from build123d import *

# Parameters (mm, degrees)
F0_R     = 33.04
F1_DEPTH = 58
F2_SIZE  = 7.62
F3_T     = -2.54
F4_R     = 2.54
F5_R     = 6
F5_W     = 10.6
F5_H     = 5
F6_DEPTH = 2.54
F7_W     = 35
F7_H     = 2.54
F8_DEPTH = 47
F9_R     = 2.54


with BuildPart() as f1:
    # F0 (on Top) → F1 (new body)
    with BuildSketch(Plane.XY):
        Circle(F0_R)
    extrude(amount=F1_DEPTH)

    # F2
    f2_edges = [f1.edges().sort_by_distance(p)[0] for p in [
        (-33.04, 0, 0),
    ]]
    chamfer(f2_edges, length=F2_SIZE)

    # F3
    f3_openings = [f1.faces().sort_by_distance(p)[0] for p in [
        (0, 0, 58),
    ]]
    offset(amount=F3_T, openings=f3_openings)

    # F4
    f4_edges = [f1.edges().sort_by_distance(p)[0] for p in [
        (-33.04, 0, 7.62),
        (-25.42, 0, 0),
    ]]
    fillet(f4_edges, radius=F4_R)

    # F5 (on face) → F6 (cut, through all)
    with BuildSketch(Plane(origin=(0, 0, 0), x_dir=(1, 0, 0), z_dir=(0, 0, -1))):
        with Locations((0, 7.62)):
            Circle(F5_R)
        with Locations((0, -6.35)):
            Rectangle(F5_W, F5_H)
    extrude(amount=-F6_DEPTH, mode=Mode.SUBTRACT)

    # F7 (on face) → F8 (join)
    with BuildSketch(Plane.XY.offset(2.54)):
        with Locations((0, 18.58)):
            Rectangle(F7_W, F7_H)
    extrude(amount=F8_DEPTH)

    # F9
    f9_edges = [f1.edges().sort_by_distance(p)[0] for p in [
        (-17.5, 18.58, 49.54),
        (17.5, 18.58, 49.54),
    ]]
    fillet(f9_edges, radius=F9_R)


solid = f1.part
Part model, mm, in its own coordinate system. A direction names the side the tool comes from. Coordinates: 2 decimals unless noted, no trailing zeros. Order: outer loops, then holes, each group sorted by start corner. A loop starts at its lowest first (then second) coordinate and runs counter-clockwise, first axis right, second up.
(1) Probe L1, parallel to Y at x = 0, z = 37; L2, parallel to X at y = 0, z = 35; L3, parallel to Y at x = 0, z = 1. List the from-to ranges inside material, lowest first.
Check sheet entries:
L1: y = -33.04 to -30.5, 17.31 to 19.85, 30.5 to 33.04
L2: x = -33.04 to -30.5, 30.5 to 33.04
L3: y = -26.42 to -13.62, -1.62 to 3.85, 8.85 to 26.42
(2) Tool access for faces 1 (the face through (0, 3.85, 1)), 2 (the face through (16.736, 18.598, 48.816)), 3 (the face through (0, 0, 0)): list every direction of +Z, -Z, +X, -X, +Y, -Y with a clear straight run to the whole face (end or side of a thin tool).
Check sheet entries:
face 1: +Z, -Z
face 2: +Z
face 3: -Z, +X, -X, +Y, -Y
(3) Pin check, flat tips, straight feed: pin 1 Ø2 at (x, y) = (-5.5, 19) entering from +Z; pin 2 Ø6 at (x, z) = (6.5, 16.5) entering from -Y; pin 3 Ø1.3 at (y, z) = (6.5, 1) entering from +X; pin 4 Ø11 at (x, y) = (0, -7.62) entering from +Z. Stop position of each tip, or through.
Check sheet entries:
pin 1: stops at z = 49.54
pin 2: stops at y = -32.85
pin 3: stops at x = 26.3
pin 4: passes through
(4) Pull direction X, two halves, no side cores. Call faces 4 (the face through (29, -10, 58)), 5 (the face through (-5.7, -25.8, 1)), 6 (the face through (0, 22, 2.54)): pulls with the +X half, pulls with the -X half, needs draft (parallel to the pull), parting line crosses it, or undercut.
Check sheet entries:
face 4: needs draft
face 5: parting line crosses it
face 6: undercut
(5) Slice it at A-A, the plane z = 46. Write the cut outline in (x, y).
Check sheet entries:
outline: circle Ø66.08 at (0, 0); (-17.5, 17.31) - (17.5, 17.31) - (17.5, 19.85) - (-17.5, 19.85) - close; hole circle Ø61 at (0, 0)
(6) Slice it at B-B, the plane x = 0. State how many separate pieces and enclosed holes the cut face has, and give its area (3 significant figures).
Check sheet entries:
separate pieces: 3
enclosed holes: 0
area: 505 mm2
